Check sheet for the modelled part. Datum: model origin and axes. Units: mm. A direction names the side the tool comes from. Round coordinates to 2 decimals unless told otherwise and drop trailing zeros. Write each loop counter-clockwise with the first axis right and the second up, starting at its lowest first coordinate (ties: lowest second). Pieces come first, ordered by that corner, then holes. Notation, with made-up numbers: (31.25, 34) - (49.25, 34) arc R19 cw to (49.25, 66) - close; hole circle Ø10 at (66.25, 45.25). An arc over 180 degrees is marked (long way). Use one line per item in the form item = value. Start each with the question number.
1) Scan lines: probe 1 along Z at (x, y) = (6.9, 38.45); probe 2 along Y at (x, z) = (3, 17); probe 3 along X at (y, z) = (28, 5.25). Record each from-to range of solid material in increasing order.
2) Section check A-A (y = 26.4). Record the boundary of the cut face in (x, z).
3) Draft check along Z on faces 3 (the face through (-0.5, 24.3, 19.8)), 4 (the face through (-1.52, 27.9, 9.97)), 5 (the face through (7, 39.6, 12)). Enter one of: +Z half, -Z half, draft (parallel to the pull), parting line (faces both ways), or undercut.
4) Set-up check for faces 1 (the face through (-1.52, 11.77, 10.35)), 2 (the face through (10, 36.6, 10)): record each of +Z, -Z, +X, -X, +Y, -Y from which the full face is reachable in a straight line by a thin tool's end or side.
5) Section check B-B (z = 9.9). Record the boundary of the cut face in (x, y), then the cut area to 3 significant figures.
6) Section check C-C (x = 6.9). Record the boundary of the cut face in (y, z), then the cut area to 3 significant figures.
7) Gauge pin test, flat ends, axial feed: P1, Ø6, axis at y = 12, z = 8.5, coming from the +X side; P2, Ø5, axis at x = 7.5, z = 10.5, coming from the -Y side. Record the tip position at first contact, or that the pin passes through.
8) Section check D-D (z = 5). Record the boundary of the cut face in (x, y), then the cut area to 3 significant figures.
from build123d import *

# Parameters (mm, degrees)
BOSS_EXTRUDE1_DEPTH = 19.8
SKETCH2_R           = 1.5
CUT_EXTRUDE1_DEPTH  = 19.8
SKETCH3_R           = 1.5
CUT_EXTRUDE2_DEPTH  = 19.8


with BuildPart() as part:
    # Sketch1 → Boss-Extrude1 (new body)
    with BuildSketch(Plane.XY):
        Polygon((0, 0), (0, 36.6), (16.8, 36.6), (16.8, 39.6), (-3, 39.6), (-3, 0), align=None)
    extrude(amount=BOSS_EXTRUDE1_DEPTH)

    # Sketch2 → Cut-Extrude1 (cut)
    with BuildSketch(Plane(origin=(0, 39.6, 0), x_dir=(1, 0, 0), z_dir=(0, 1, 0))):
        with Locations(Location((6.9, -9.9, 0), (0, 0, 180))):
            Circle(SKETCH2_R)
    extrude(amount=-CUT_EXTRUDE1_DEPTH, mode=Mode.SUBTRACT)

    # Sketch3 → Cut-Extrude2 (cut)
    with BuildSketch(Plane.ZY.offset(3)):
        with Locations(Location((9.9, 26.4, 0), (0, 0, 270))):
            Circle(SKETCH3_R)
        with Locations(Location((9.9, 13.2, 0), (0, 0, 270))):
            Circle(SKETCH3_R)
    extrude(amount=-CUT_EXTRUDE2_DEPTH, mode=Mode.SUBTRACT)


solid = part.part
Results are:
q1.probe_1 = 0 to 8.4, 11.4 to 19.8
q1.probe_2 = 36.6 to 39.6
q1.probe_3 = -3 to 0
q2.outline = (-3, 0) - (0, 0) - (0, 8.4) - (-3, 8.4) - close; (-3, 11.4) - (0, 11.4) - (0, 19.8) - (-3, 19.8) - close
q3.face_3 = +Z half
q3.face_4 = undercut
q3.face_5 = draft
q4.face_1 = +X, -X
q4.face_2 = +Z, -Z, +X, -Y
q5.outline = (-3, 0) - (0, 0) - (0, 11.7) - (-3, 11.7) - close; (-3, 14.7) - (0, 14.7) - (0, 24.9) - (-3, 24.9) - close; (-3, 27.9) - (0, 27.9) - (0, 36.6) - (5.4, 36.6) - (5.4, 39.6) - (-3, 39.6) - close; (8.4, 36.6) - (16.8, 36.6) - (16.8, 39.6) - (8.4, 39.6) - close
q5.area = 142 mm²
q6.outline = (36.6, 0) - (39.6, 0) - (39.6, 8.4) - (36.6, 8.4) - close; (36.6, 11.4) - (39.6, 11.4) - (39.6, 19.8) - (36.6, 19.8) - close
q6.area = 50.4 mm²
q7.P1 = 0
q7.P2 = 36.6
q8.outline = (-3, 0) - (0, 0) - (0, 36.6) - (16.8, 36.6) - (16.8, 39.6) - (-3, 39.6) - close
q8.area = 169 mm²
